Geometry: final body of the model. Coordinates: model frame, mm. A direction names the side the tool comes from. Coordinates: 2 decimals unless noted, no trailing zeros. Order: outer loops, then holes, each group sorted by start corner. A loop starts at its lowest first (then second) coordinate and runs counter-clockwise, first axis right, second up. Notation, with made-up numbers: (87.25, 33.5) -> (112.25, 33.5) arc R35 cw to (112.25, 69.5) -> close; hole circle Ø5 at (-39, -30). An arc over 180 degrees is marked (long way). Use one line per item in the form item = value.
```python
from build123d import *

# Parameters (mm, degrees)
SKETCH1_W           = 5
SKETCH1_H           = 18
BOSS_EXTRUDE1_DEPTH = 1
SKETCH2_R           = 1.5
SKETCH2_W           = 3
SKETCH2_H           = 2
CUT_EXTRUDE1_DEPTH  = 10.394147114


with BuildPart() as part:
    # Sketch1 → Boss-Extrude1 (new body)
    with BuildSketch(Plane.XY):
        Rectangle(SKETCH1_W, SKETCH1_H)
    extrude(amount=BOSS_EXTRUDE1_DEPTH)

    # Sketch2 → Cut-Extrude1 (cut, through all)
    with BuildSketch(Plane.XY.offset(1)):
        with Locations((0, 5)):
            Circle(SKETCH2_R)
        with Locations(Location((0, -5, 0), (0, 0, 180))):
            Circle(SKETCH2_R)
        with Locations((1, 0)):
            Rectangle(SKETCH2_W, SKETCH2_H)
    extrude(amount=-CUT_EXTRUDE1_DEPTH, mode=Mode.SUBTRACT)


solid = part.part
```
1) Section C-C, the plane x = 1.95. Output: boundary loops of the cut face in (y, z), and give its area (3 significant figures).
Results found:
outline = (-9, 0) -> (-1, 0) -> (-1, 1) -> (-9, 1) -> close; (1, 0) -> (9, 0) -> (9, 1) -> (1, 1) -> close
area = 16.0 mm2
2) Contact query for a flat-ended pin moving along its axis: P1, Ø1.8, axis at x = 0, y = -5, coming from the -Z side. Output: stop coordinate, or through.
Results found:
P1 = through
3) Section D-D, the plane z = 0.2. Output: boundary loops of the cut face in (x, y), and give its area (3 significant figures).
Results found:
outline = (-2.5, -9) -> (2.5, -9) -> (2.5, -1) -> (-0.5, -1) -> (-0.5, 1) -> (2.5, 1) -> (2.5, 9) -> (-2.5, 9) -> close; hole circle Ø3 at (0, -5); hole circle Ø3 at (0, 5)
area = 69.9 mm2
4) Pull-direction query (Y, two-part tool) for faces 1 (the flat face through (1, -1, 0.5)), 2 (the flat face through (0, 9, 0.5)), 3 (the flat face through (-1, 0, 0)), 4 (the cylindrical face through (-1.5, 5.07, 0.51)); classes: released by +Y, released by -Y, zero draft, split by the parting line, or undercut.
Results found:
face_1 = undercut
face_2 = released by +Y
face_3 = zero draft
face_4 = undercut
5) Access query for faces 5 (the flat face through (0, -9, 0.5)), 6 (the flat face through (1, 1, 0.5)). Directions: +Z, -Z, +X, -X, +Y, -Y. A direction counts if a zero-diameter tool reaches every point of the face in a straight line with its end or side. Return the directions, or none.
Results found:
face_5 = +Z, -Z, +X, -X, -Y
face_6 = +Z, -Z, +X
6) Section B-B, the plane x = 0. Output: boundary loops of the cut face in (y, z), and give its area (3 significant figures).
Results found:
outline = (-9, 0) -> (-6.5, 0) -> (-6.5, 1) -> (-9, 1) -> close; (-3.5, 0) -> (-1, 0) -> (-1, 1) -> (-3.5, 1) -> close; (1, 0) -> (3.5, 0) -> (3.5, 1) -> (1, 1) -> close; (6.5, 0) -> (9, 0) -> (9, 1) -> (6.5, 1) -> close
area = 10.0 mm2
7) Material intervals for probe 1 along Y at (x, z) = (0, 0.5); probe 2 along X at (y, z) = (-5, 0.7); probe 3 along Y at (x, z) = (1.65, 0.2), sorted ascending. Write a range as from..to.
Results found:
probe_1 = -9..-6.5, -3.5..-1, 1..3.5, 6.5..9
probe_2 = -2.5..-1.5, 1.5..2.5
probe_3 = -9..-1, 1..9
8) Section A-A, the plane y = -5. Output: boundary loops of the cut face in (x, z).
Results found:
outline = (-2.5, 0) -> (-1.5, 0) -> (-1.5, 1) -> (-2.5, 1) -> close; (1.5, 0) -> (2.5, 0) -> (2.5, 1) -> (1.5, 1) -> close
